from build123d import *

# Parameters (mm, degrees)
SKETCH1_W           = 9.525
SKETCH1_H           = 10.795
BOSS_EXTRUDE1_DEPTH = 0.889
SKETCH2_W           = 7.112
SKETCH2_H           = 1.143
CUT_EXTRUDE1_DEPTH  = 1.27
LPATTERN1_COUNT     = 4
LPATTERN1_PITCH     = 2.54
SWEEP1_START        = 3.302
SWEEP1_DEPTH        = 1.016
LPATTERN2_COUNT     = 4
LPATTERN2_PITCH     = 2.54
CUT_EXTRUDE2_DEPTH  = 12.8580274
FILLET2_R           = 0.127


# Read off the part's stored shape, not the designer's step: Sweep1
with BuildPart() as part:
    # Sketch1 → Boss-Extrude1 (new, symmetric)
    with BuildSketch(Plane.XY):
        Rectangle(SKETCH1_W, SKETCH1_H)
    extrude(amount=BOSS_EXTRUDE1_DEPTH, both=True)

    # Sketch2 → Cut-Extrude1 (cut)
    with BuildSketch(Plane.XY.offset(0.889)):
        with Locations((-1.2065, 3.81)):
            Rectangle(SKETCH2_W, SKETCH2_H)
    cut_extrude1 = extrude(amount=-CUT_EXTRUDE1_DEPTH, mode=Mode.SUBTRACT)

    # LPattern1: Cut-Extrude1 ×4
    with Locations(*[(0, -i * LPATTERN1_PITCH, 0) for i in range(1, LPATTERN1_COUNT)]):
        add(cut_extrude1, mode=Mode.SUBTRACT)

    # Sweep1 outline → Sweep1 (add)
    with BuildSketch(Plane(origin=(0, 0, 0), x_dir=(1, 0, 0), z_dir=(0, 1, 0)).offset(SWEEP1_START)):
        with BuildLine():
            add(Edge.make_bspline(
                [(-2.958664485, 0.03175), (-2.706405798, -0.084396657), (-2.195293689, -0.319726362), (-1.514674501, -0.811036045), (-0.723468732, -1.093477281), (0.111091297, -1.1480463), (0.950883413, -0.99405052), (1.715489301, -0.68557292), (2.154910348, -0.386399802), (2.3495, -0.248288405)],
                knots=[0, 0, 0, 0, 0.1400972, 0.283856925, 0.421522391, 0.557109715, 0.701349819, 0.849245032, 0.969367335, 0.969367335, 0.969367335, 0.969367335], degree=3))
            Line((-2.958664485, 0.03175), (-4.7625, 0.03175))
            Line((-4.7625, 0.03175), (-4.7625, -0.03175))
            Line((-4.7625, -0.03175), (-2.968725914, -0.03175))
            add(Edge.make_bspline(
                [(-2.968725914, -0.03175), (-2.714491455, -0.15140088), (-2.19937615, -0.393830641), (-1.50930601, -0.887085656), (-0.710525949, -1.159958237), (0.131263589, -1.2104677), (0.978085908, -1.052203574), (1.73427594, -0.74581201), (2.165863748, -0.455666821), (2.3495, -0.326036057)],
                knots=[0, 0, 0, 0, 0.1400972, 0.283856925, 0.421522391, 0.557109715, 0.701349819, 0.849245032, 0.961516171, 0.961516171, 0.961516171, 0.961516171], degree=3))
            Line((2.3495, -0.326036057), (2.3495, -0.248288405))
        make_face()
    sweep1 = extrude(amount=SWEEP1_DEPTH)

    # LPattern2: Sweep1 ×4
    with Locations(*[(0, -i * LPATTERN2_PITCH, 0) for i in range(1, LPATTERN2_COUNT)]):
        add(sweep1)

    # Sketch5 → Cut-Extrude2 (cut, through all)
    with BuildSketch(Plane.XZ.offset(5.3975)):
        with BuildLine():
            Line((4.1275, 0.889), (4.830136411, 0.889))
            Line((4.830136411, 0.889), (4.830136411, -0.889))
            Line((4.830136411, -0.889), (4.1275, -0.889))
            ThreePointArc((4.1275, -0.889), (4.576512806, -0.703012806), (4.7625, -0.254))
            Line((4.7625, -0.254), (4.7625, 0.254))
            ThreePointArc((4.7625, 0.254), (4.576512806, 0.703012806), (4.1275, 0.889))
        make_face()
    extrude(amount=-CUT_EXTRUDE2_DEPTH, mode=Mode.SUBTRACT)

    # Fillet2
    fillet2_edges = [part.edges().sort_by_distance(p)[0] for p in [
        (-0.3175, -5.3975, 0.889),
        (-0.3175, 5.3975, -0.889),
        (-0.3175, 5.3975, 0.889),
        (4.7625, -5.3975, 0),
        (4.7625, 5.3975, 0),
        (4.576512806, -5.3975, 0.703012806),
        (4.576512806, -5.3975, -0.703012806),
        (4.576512806, 5.3975, -0.703012806),
        (4.576512806, 5.3975, 0.703012806),
        (-0.3175, -5.3975, -0.889),
    ]]
    fillet(fillet2_edges, radius=FILLET2_R)


solid = part.part
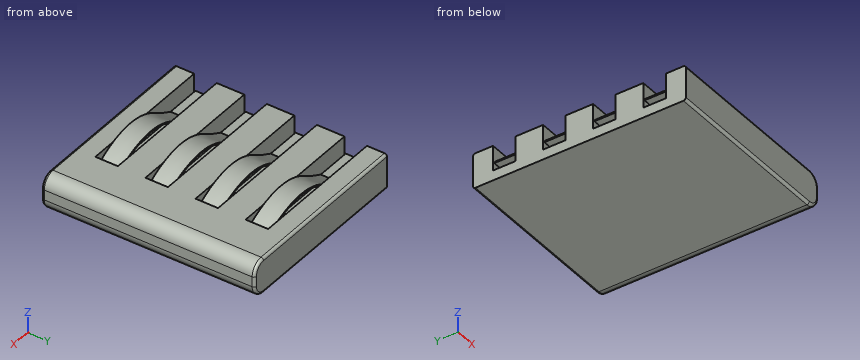
For this review, take the finished solid that the model builds, in its own axes (mm). Round coordinates to 2 decimals unless told otherwise and drop trailing zeros. Order: outer loops, then holes, each group sorted by start corner. A loop starts at its lowest first (then second) coordinate and runs counter-clockwise, first axis right, second up. Notation, with made-up numbers: (48.5, -25.75) -> (87.5, -25.75) arc R24 cw to (87.5, -2.75) -> close; hole circle Ø6 at (60.5, -24). An arc over 180 degrees is marked (long way). Put each result on its own line as item: value.
Q1. Add section A-A on y = -3. Write out the cut boundary in (x, z) (1 decimal), plus the area to 3 significant figures.
Check result:
outline: (-4.8, -0.9) -> (4.1, -0.9) arc R0.6 ccw to (4.8, -0.3) -> (4.8, 0.3) arc R0.6 ccw to (4.1, 0.9) -> (-4.8, 0.9) -> close
area: 16.8 mm2
Q2. For probe 1 along Y at (x, z) = (-4, 0.7); probe 2 along X at (y, z) = (1.25, -0.3); probe 3 along Z at (x, y) = (-2.75, -2.5), list the stretches that pass through material, from the lowest coordinate up. Write a range as [from, to].
Check result:
probe 1: [-5.4, -4.38], [-3.24, -1.84], [-0.7, 0.7], [1.84, 3.24], [4.38, 5.4]
probe 2: [2.35, 4.76]
probe 3: [-0.89, 0.89]
Q3. Add section B-B on x = 3. Write out the cut boundary in (y, z).
Check result:
outline: (-5.4, -0.76) arc R0.13 ccw to (-5.27, -0.89) -> (5.27, -0.89) arc R0.13 ccw to (5.4, -0.76) -> (5.4, 0.76) arc R0.13 ccw to (5.27, 0.89) -> (-5.27, 0.89) arc R0.13 ccw to (-5.4, 0.76) -> close
Q4. Add section C-C on x = 1.25. State how many separate pieces and enclosed holes the cut face has, plus the area to 3 significant figures.
Check result:
separate pieces: 5
enclosed holes: 0
area: 13.6 mm2
Q5. Insertion check: pin 1 Ø0.8 at (x, y) = (-3.5, -3.5) entering from +Z; pin 2 Ø0.5 at (x, y) = (-4, 4) entering from +Z; pin 3 Ø0.6 at (x, y) = (-0.5, -4) entering from +Z; pin 4 Ø1 at (y, z) = (4, 0.5) entering from -X. Each pin has a flat end and moves straight along its axis. Give the tip position at first contact, or say it passes through.
Check result:
pin 1: z = 0.89
pin 2: z = 0.03
pin 3: z = 1.18
pin 4: x = -4.76
